Build history of the part. All positions in model axes, mm. A direction names the side the tool comes from. Round coordinates to 2 decimals unless told otherwise and drop trailing zeros. Write each loop counter-clockwise with the first axis right and the second up, starting at its lowest first coordinate (ties: lowest second). Pieces come first, ordered by that corner, then holes. Notation, with made-up numbers: (78, 4) -> (110, 4) arc R15 cw to (110, 26) -> close; hole circle Ø3 at (27, 17). An arc over 180 degrees is marked (long way). Answer in a Markdown table with one row per item.
Autodesk Inventor part; units mm, degrees
ref_plane "YZ Plane" through (0, 0, 0) normal (1, 0, 0) x (0, 1, 0)
ref_plane "XZ Plane" through (0, 0, 0) normal (0, 1, 0) x (-1, 0, 0)
ref_plane "XY Plane" through (0, 0, 0) normal (0, 0, 1) x (1, 0, 0)
sketch "Sketch1" plane through (0, 0, 0) normal (0, 1, 0) x (-1, 0, 0)
  circle A0 centre (0, 0) radius 5.461
  dimension "d0" = 10.922
extrude "Extrusion1" add sketch "Sketch1" along normal blind 20.066
sketch "Sketch2" plane through (0, 0, 0) normal (1, 0, 0) x (0, 1, 0)
  line L0 (2.7178, -0.3105) -> (7.8486, -0.3105)
  line L1 (7.8486, -0.3105) -> (7.8486, -9.4037)
  line L2 (7.8486, -9.4037) -> (2.7178, -9.4037)
  line L3 (2.7178, -9.4037) -> (2.7178, -0.3105)
  line L4 (0, 5.461) -> (0, -5.461)
  line L5 (20.066, -5.461) -> (20.066, 5.461)
  point P0 (0, 0)
  dimension "d3" = 9.0932
  dimension "d4" = 2.7178
  dimension "d12" = 12.2174
revolve "Revolution1" add sketch "Sketch2" angle 360 about axis through (0, 2.7178, -0.3105) along (0, 1, 0)
sketch "Sketch3" plane through (0, 0, 0) normal (0, -1, 0) x (1, 0, 0)
  circle A0 centre (0, 0) radius 5.461
  circle A1 centre (0, 0) radius 4.8747
extrude "Extrusion2" add sketch "Sketch3" along normal blind 5.08 contours A1
sketch "Sketch4" plane through (0, 20.066, 0) normal (0, 1, 0) x (1, 0, 0)
  circle A0 centre (0, 0) radius 5.461
  circle A1 centre (0, 0) radius 3.81
  dimension "d9" = 7.62
extrude "Extrusion3" cut sketch "Sketch4" against normal blind 5.588 contours A1
properties part number "SmallConnector"
Q1. Saw through at C-C on z = -4.5. Write the cut outline in (x, y), plus the area to 3 significant figures.
A:
| item | result |
|---|---|
| outline | (-8.07, 2.72) -> (-3.09, 2.72) -> (-3.09, 0) -> (-1.87, 0) -> (-1.87, -5.08) -> (1.87, -5.08) -> (1.87, 0) -> (3.09, 0) -> (3.09, 2.72) -> (8.07, 2.72) -> (8.07, 7.85) -> (3.09, 7.85) -> (3.09, 20.07) -> (-3.09, 20.07) -> (-3.09, 7.85) -> (-8.07, 7.85) -> close |
| area | 194 mm² |
Q2. Drop flat-ended pins along their axis: P1, Ø8, axis at y = 4, z = 4, coming from the -X side; P2, Ø2, axis at x = -2, z = -6.5, coming from the -Y side; P3, Ø6, axis at x = 0.5, z = -0.5, coming from the +Y side. Give the stop position or say it passes through.
A:
| item | result |
|---|---|
| P1 | x = -9.09 |
| P2 | y = 2.72 |
| P3 | y = 14.48 |
Q3. Saw through at D-D on y = 15. Write the cut outline in (x, z).
A:
| item | result |
|---|---|
| outline | circle Ø10.92 at (0, 0); hole circle Ø7.62 at (0, 0) |
Q4. Wall check: line 1 (Z direction, x = 0, y = 18.55); line 2 (Y direction, x = -3.5, z = -4). Give the ranges that are in metal, low to high. Write a range as [from, to].
A:
| item | result |
|---|---|
| line 1 | [-5.46, -3.81], [3.81, 5.46] |
| line 2 | [0, 20.07] |
Q5. Saw through at A-A on x = 0. Write the cut outline in (y, z).
A:
| item | result |
|---|---|
| outline | (-5.08, -4.87) -> (0, -4.87) -> (0, -5.46) -> (2.72, -5.46) -> (2.72, -9.4) -> (7.85, -9.4) -> (7.85, -5.46) -> (20.07, -5.46) -> (20.07, -3.81) -> (14.48, -3.81) -> (14.48, 3.81) -> (20.07, 3.81) -> (20.07, 5.46) -> (7.85, 5.46) -> (7.85, 8.78) -> (2.72, 8.78) -> (2.72, 5.46) -> (0, 5.46) -> (0, 4.87) -> (-5.08, 4.87) -> close |
Q6. Two-plate mould, pull along X, no slides. Class faces 1 (the flat face through (0, -5.08, 0)), 2 (the cylindrical face through (-0.83, 17.31, 3.72)), 3 (the cylindrical face through (-5.21, 13.87, -1.64)): released by +X, released by -X, zero draft, split by the parting line, or undercut.
A:
| item | result |
|---|---|
| face 1 | zero draft |
| face 2 | undercut |
| face 3 | split by the parting line |
Q7. Which spindle directions (+Z, -Z, +X, -X, +Y, -Y) get a long thin tool onto all of the face, cutting with end or side? Do faces 4 (the flat face through (-1, 20.066, 4)), 5 (the flat face through (4, 7.849, -4)), 6 (the flat face through (4, 2.718, -4)). Say none if no direction does.
A:
| item | result |
|---|---|
| face 4 | +Z, -Z, +X, -X, +Y |
| face 5 | +Y |
| face 6 | -Y |
Q8. Saw through at B-B on y = 9.25. Write the cut outline in (x, z), plus the area to 3 significant figures.
A:
| item | result |
|---|---|
| outline | circle Ø10.92 at (0, 0) |
| area | 93.7 mm² |
